For this review, take the finished solid that the model builds, in its own axes (mm). Face numbers are marked on the shaded views. A direction names the side the tool comes from. Round coordinates to 2 decimals unless told otherwise and drop trailing zeros. Write each loop counter-clockwise with the first axis right and the second up, starting at its lowest first coordinate (ties: lowest second). Pieces come first, ordered by that corner, then holes. Notation, with made-up numbers: (6.25, 15.5) -> (36.25, 15.5) arc R19 cw to (36.25, 50.5) -> close; hole circle Ø9 at (36.5, 15). An arc over 180 degrees is marked (long way). Answer in a Markdown table with one row per item.
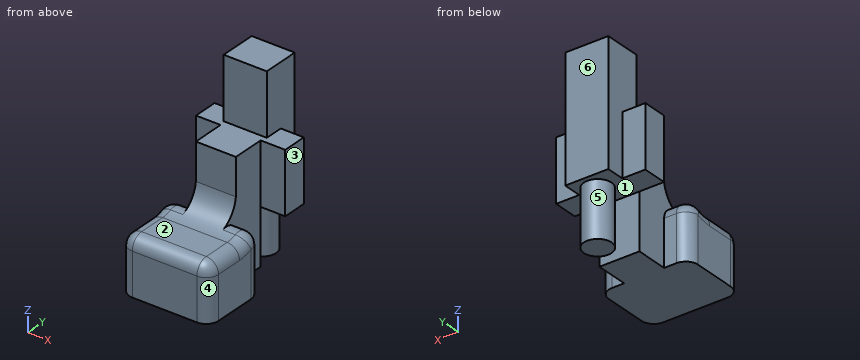
from build123d import *

# Parameters (mm, degrees)
BOSS_EXTRUDE1_DEPTH = 10
SKETCH3_W           = 14.5
SKETCH3_H           = 11
CUT_EXTRUDE2_DEPTH  = 2
BOSS_EXTRUDE2_DEPTH = 10
SKETCH2_R           = 2.25
BOSS_EXTRUDE4_DEPTH = 9
CUT_EXTRUDE5_DEPTH  = 28.596014205
FILLET1_R           = 2


with BuildPart() as part:
    # Sketch1 → Boss-Extrude1 (new body)
    with BuildSketch(Plane.XY):
        Polygon((2.75, 0), (2.75, 5.3), (6.75, 5.3), (6.75, 9.3), (3, 9.3), (3, 12.3), (-4, 12.3), (-4, 9.3), (-7.75, 9.3), (-7.75, 5.3), (-3.75, 5.3), (-3.75, 0), (-7.75, 0), (-7.75, -11), (6.75, -11), (6.75, 0), align=None)
    extrude(amount=BOSS_EXTRUDE1_DEPTH)

    # Sketch3 → Cut-Extrude2 (cut)
    with BuildSketch(Plane.XY.offset(10)):
        with Locations((-0.5, -5.5)):
            Rectangle(SKETCH3_W, SKETCH3_H)
    extrude(amount=-CUT_EXTRUDE2_DEPTH, mode=Mode.SUBTRACT)

    # Sketch4 → Boss-Extrude2 (add)
    with BuildSketch(Plane.XY.offset(10)):
        Polygon((3, 9.3), (3, 12.3), (-4, 12.3), (-4, 9.3), (-4, 6.3), (3, 6.3), align=None)
    extrude(amount=BOSS_EXTRUDE2_DEPTH)

    # Sketch2 → Boss-Extrude4 (add)
    with BuildSketch(Plane(origin=(0, 0, 0), x_dir=(-1, 0, 0), z_dir=(0, 0, -1))):
        with Locations((0, 9.3)):
            Circle(SKETCH2_R)
        Polygon((-2.75, 0), (-2.75, 5.3), (3.75, 5.3), (3.75, 0), (7.75, 0), (7.75, -11), (-6.75, -11), (-6.75, 0), align=None)
    extrude(amount=BOSS_EXTRUDE4_DEPTH)

    # Sketch6 → Cut-Extrude5 (cut, through all)
    with BuildSketch(Plane(origin=(6.75, 0, 0), x_dir=(0, 0, -1), z_dir=(1, 0, 0))):
        with BuildLine():
            Line((-4, 0), (-8, 0))
            Line((-8, 0), (-8, -11))
            Line((-8, -11), (0.027692569, -11))
            Line((0.027692569, -11), (0.027692569, -4.5))
            ThreePointArc((0.027692569, -4.5), (-1.12628941, -1.480384651), (-4, 0))
        make_face()
    extrude(amount=-CUT_EXTRUDE5_DEPTH, mode=Mode.SUBTRACT)

    # Fillet1
    fillet1_edges = [part.edges().sort_by_distance(p)[0] for p in [
        (6.75, 0, -2.5),
        (6.75, -11, -4.513846285),
        (-7.75, -11, -4.513846285),
        (-7.75, 0, -2.5),
        (6.75, -1.480384651, 1.12628941),
        (-5.75, 0, 4),
        (4.75, 0, 4),
        (6.75, -7.75, -0.027692569),
        (-0.5, -11, -0.027692569),
        (-7.75, -1.480384651, 1.12628941),
        (-7.75, -7.75, -0.027692569),
    ]]
    fillet(fillet1_edges, radius=FILLET1_R)


solid = part.part
1) For the marked faces 1, 2 and 3, list the 3-axis set-ups (+Z, -Z, +X, -X, +Y, -Y) from which the entire face can be reached by the end or side of a thin tool; tool diameter is ignored.
Solved:
| item | result |
|---|---|
| face 1 | -Z |
| face 2 | +Z, +X, -X, -Y |
| face 3 | +Z, -Z, +X, +Y, -Y |
2) For line 1 (Y direction, x = -4.75, z = 2.25); line 2 (Y direction, x = 0, z = 15.25); line 3 (Z direction, x = -2.5, y = 9.5), list the stretches that pass through material, from the lowest coordinate up. Write a range as [from, to].
Solved:
| item | result |
|---|---|
| line 1 | [5.3, 9.3] |
| line 2 | [6.3, 12.3] |
| line 3 | [0, 20] |
3) Consider section B-B on z = 3. State the section outline as (x, y) points, then the cut area to 3 significant figures.
Solved:
| item | result |
|---|---|
| outline | (-7.75, 5.3) -> (-3.75, 5.3) -> (-3.75, -0.23) -> (2.75, -0.23) -> (2.75, 5.3) -> (6.75, 5.3) -> (6.75, 9.3) -> (3, 9.3) -> (3, 12.3) -> (-4, 12.3) -> (-4, 9.3) -> (-7.75, 9.3) -> close |
| area | 115 mm² |
4) Mouldability with a two-part tool opening along Y and no side actions: class the marked faces 4, 5 and 6 as pulls with the +Y half, pulls with the -Y half, needs draft (parallel to the pull), parting line crosses it, or undercut.
Solved:
| item | result |
|---|---|
| face 4 | pulls with the -Y half |
| face 5 | undercut |
| face 6 | pulls with the +Y half |
5) Consider section D-D on x = 0. State the section outline as (y, z) points.
Solved:
| item | result |
|---|---|
| outline | (-11, -9) -> (5.3, -9) -> (5.3, 0) -> (7.05, 0) -> (7.05, -9) -> (11.55, -9) -> (11.55, 0) -> (12.3, 0) -> (12.3, 20) -> (6.3, 20) -> (6.3, 10) -> (0, 10) -> (0, 4) arc R4.53 cw to (-4.5, -0.03) -> (-9, -0.03) arc R2 ccw to (-11, -2.03) -> close |
6) Consider section C-C on y = 2.5. State the section outline as (x, z) points.
Solved:
| item | result |
|---|---|
| outline | (-3.75, -9) -> (2.75, -9) -> (2.75, 10) -> (-3.75, 10) -> close |
7) Clearance check with flat-ended pins moving along their axes: pin 1 Ø2 at (x, z) = (4.5, 3.5) entering from -Y; pin 2 Ø3.5 at (x, z) = (0.5, 14.5) entering from -Y; pin 3 Ø1.9 at (x, z) = (4.5, 7.5) entering from +Y. State where each tip first meets the part, or that it passes through.
Solved:
| item | result |
|---|---|
| pin 1 | y = 5.3 |
| pin 2 | y = 6.3 |
| pin 3 | y = 9.3 |
8) Consider section A-A on x = 5.5. State the section outline as (y, z) points.
Solved:
| item | result |
|---|---|
| outline | (-10.85, -9) -> (-0.15, -9) -> (-0.15, -1.53) arc R1.85 ccw to (-2.71, 0.18) arc R4.67 cw to (-4.5, -0.17) -> (-9, -0.17) arc R1.85 ccw to (-10.85, -2.03) -> close; (5.3, 0) -> (9.3, 0) -> (9.3, 10) -> (5.3, 10) -> close |
